Geometry check sheet. Reference: the model listing, model coordinates, mm. A direction names the side the tool comes from. Give positions to 0.01 mm unless a question says otherwise; leave off trailing zeros. Order: outer loops, then holes, each group sorted by start corner. A loop starts at its lowest first (then second) coordinate and runs counter-clockwise, first axis right, second up. Notation, with made-up numbers: M 21.5,6 L 48.5,6 A16 ccw 48.5,37 Z; hole C 46,66.25 d9. An arc over 180 degrees is marked long. Answer as CSV lines item,"result". Start each with the question number.
Q1. Set-up check for faces 1 (the flat face through (0, 3, 25)), 2 (the cylindrical face through (37.43, 0.6, -0.35)): record each of +Z, -Z, +X, -X, +Y, -Y from which the full face is reachable in a straight line by a thin tool's end or side.
Q2. Go/stop test with a flat-tipped pin: pin 1 (6 mm diameter, centred on x = -9, z = 21, fed in from +Y). Record where the tip stops, or that it passes through.
Q3. Section check D-D, the plane z = 0.5. Record the boundary of the cut face in (x, y), then the cut area to 3 significant figures.
Q4. Thickness scan on line 1 (X direction, y = 2.7, z = -23); line 2 (X direction, y = 3.25, z = -16); line 3 (Z direction, x = -3.5, y = 2.7). Record the ranges inside material, lowest first.
Q5. Section check C-C, the plane x = 25. Record the boundary of the cut face in (y, z), then the cut area to 3 significant figures.
Q6. Mould release check, pull along X, two halves, no side actions. Record for faces 3 (the cylindrical face through (37.43, 3.01, -26.4)), 4 (the cylindrical face through (0.5, 0.6, -26.43)), 5 (the flat face through (-1, 2, 0)): +X half, -X half, draft (parallel to the pull), parting line (faces both ways), or undercut.
Q7. Section check A-A, the plane z = -23. Record the boundary of the cut face in (x, y).
Q8. Section check B-B, the plane x = -34. Record the boundary of the cut face in (y, z), then the cut area to 3 significant figures.
```python
from build123d import *

# Parameters (mm, degrees)
SCHIZZO1_W                   = 76
SCHIZZO1_H                   = 54
ESTRUSIONE_ESTRUSIONE1_DEPTH = 4
SCHIZZO2_W                   = 72
SCHIZZO2_H                   = 50
TAGLIO_ESTRUSIONE1_DEPTH     = 2
SCHIZZO3_R                   = 3.65
SCHIZZO3_R_2                 = 1.65
ESTRUSIONE_ESTRUSIONE2_DEPTH = 2
SCHIZZO3_11_R                = 1.65
TAGLIO_ESTRUSIONE4_DEPTH     = 47.658332589
SCHIZZO5_R                   = 11
TAGLIO_ESTRUSIONE5_DEPTH     = 2
RACCORDO1_R                  = 2
RACCORDO2_R                  = 1


with BuildPart() as part:
    # Schizzo1 → Estrusione-Estrusione1 (new body)
    with BuildSketch(Plane(origin=(0, 0, 0), x_dir=(1, 0, 0), z_dir=(0, 1, 0))):
        Rectangle(SCHIZZO1_W, SCHIZZO1_H)
    extrude(amount=ESTRUSIONE_ESTRUSIONE1_DEPTH)

    # Schizzo2 → Taglio-Estrusione1 (cut)
    with BuildSketch(Plane(origin=(0, 4, 0), x_dir=(1, 0, 0), z_dir=(0, 1, 0))):
        Rectangle(SCHIZZO2_W, SCHIZZO2_H)
    extrude(amount=-TAGLIO_ESTRUSIONE1_DEPTH, mode=Mode.SUBTRACT)

    # Schizzo3 → Estrusione-Estrusione2 (add)
    # profile 1 of 4: a face of its own
    with BuildSketch(Plane(origin=(0, 2, 0), x_dir=(1, 0, 0), z_dir=(0, 1, 0))):
        with Locations((34, 23)):
            Circle(SCHIZZO3_R)
        with Locations(Location((34, 23, 0), (0, 0, 270))):
            Circle(SCHIZZO3_R_2, mode=Mode.SUBTRACT)
    # profile 2 of 4: a face of its own
    with BuildSketch(Plane(origin=(0, 2, 0), x_dir=(1, 0, 0), z_dir=(0, 1, 0))):
        with Locations((-34, 23)):
            Circle(SCHIZZO3_R)
        with Locations(Location((-34, 23, 0), (0, 0, 270))):
            Circle(SCHIZZO3_R_2, mode=Mode.SUBTRACT)
    # profile 3 of 4: a face of its own
    with BuildSketch(Plane(origin=(0, 2, 0), x_dir=(1, 0, 0), z_dir=(0, 1, 0))):
        with Locations((34, -23)):
            Circle(SCHIZZO3_R)
        with Locations(Location((34, -23, 0), (0, 0, 270))):
            Circle(SCHIZZO3_R_2, mode=Mode.SUBTRACT)
    # profile 4 of 4: a face of its own
    with BuildSketch(Plane(origin=(0, 2, 0), x_dir=(1, 0, 0), z_dir=(0, 1, 0))):
        with Locations((-34, -23)):
            Circle(SCHIZZO3_R)
        with Locations(Location((-34, -23, 0), (0, 0, 270))):
            Circle(SCHIZZO3_R_2, mode=Mode.SUBTRACT)
    extrude(amount=ESTRUSIONE_ESTRUSIONE2_DEPTH)

    # Schizzo3<11> → Taglio-Estrusione4 (cut, through all)
    with BuildSketch(Plane(origin=(0, 2, 0), x_dir=(1, 0, 0), z_dir=(0, 1, 0))):
        with Locations(Location((-34, 23, 0), (0, 0, 270))):
            Circle(SCHIZZO3_11_R)
        with Locations(Location((-34, -23, 0), (0, 0, 270))):
            Circle(SCHIZZO3_11_R)
        with Locations(Location((34, -23, 0), (0, 0, 270))):
            Circle(SCHIZZO3_11_R)
        with Locations(Location((34, 23, 0), (0, 0, 270))):
            Circle(SCHIZZO3_11_R)
    extrude(amount=-TAGLIO_ESTRUSIONE4_DEPTH, mode=Mode.SUBTRACT)

    # Schizzo5 → Taglio-Estrusione5 (cut)
    with BuildSketch(Plane.XZ):
        with Locations(Location((25, 8, 0), (0, 0, 270))):
            Circle(SCHIZZO5_R)
    extrude(amount=-TAGLIO_ESTRUSIONE5_DEPTH, mode=Mode.SUBTRACT)

    # Raccordo1
    raccordo1_edges = [part.edges().sort_by_distance(p)[0] for p in [
        (0, 0, 27),
        (-38, 0, 0),
        (0, 0, -27),
        (38, 0, 0),
        (38, 2, 27),
        (-38, 2, 27),
        (-38, 2, -27),
        (38, 2, -27),
    ]]
    fillet(raccordo1_edges, radius=RACCORDO1_R - 0.0001)  # a hair under: the kernel refuses the full size

    # Raccordo2
    raccordo2_edges = [part.edges().sort_by_distance(p)[0] for p in [
        (30.946723072, 3, -25),
        (36, 3, -19.946723072),
        (-36, 3, -19.946723072),
        (-30.946723072, 3, -25),
        (-30.946723072, 3, 25),
        (-36, 3, 19.946723072),
        (36, 3, 19.946723072),
        (30.946723072, 3, 25),
    ]]
    fillet(raccordo2_edges, radius=RACCORDO2_R)


solid = part.part
```
Answer block:
1,face 1,"+Y"
1,face 2,"+Z, -Z, +X, -Y"
2,pin 1,"stops at y = 2"
3,outline,"M -38,2 A2 ccw -36,0 L 16.95,0 L 16.95,2 L -36,2 L -36,4 L -38,4 Z; M 33.05,0 L 36,0 A2 ccw 38,2 L 38,4 L 36,4 L 36,2 L 33.05,2 Z"
3,area,"126 mm2"
4,line 1,"x = -38 to -35.65, -32.35 to -30.35, 30.35 to 32.35, 35.65 to 38"
4,line 2,"x = -38 to -36, 36 to 38"
4,line 3,"z = -27 to -25, 25 to 27"
5,outline,"M 0,-25 A2 ccw 2,-27 L 4,-27 L 4,-25 L 2,-25 L 2,-3 L 0,-3 Z; M 0,19 L 2,19 L 2,25 L 4,25 L 4,27 L 2,27 A2 ccw 0,25 Z"
5,area,"70.3 mm2"
6,face 3,"+X half"
6,face 4,"draft"
6,face 5,"undercut"
7,outline,"M -38,2 A2 ccw -36,0 L -35.65,0 L -35.65,4 L -38,4 Z; M -32.35,0 L 32.35,0 L 32.35,4 L 30.35,4 L 30.35,2 L -30.35,2 L -30.35,4 L -32.35,4 Z; M 35.65,0 L 36,0 A2 ccw 38,2 L 38,4 L 35.65,4 Z"
8,outline,"M 0,-25 A2 ccw 2,-27 L 4,-27 L 4,-24.65 L 0,-24.65 Z; M 0,-21.35 L 4,-21.35 L 4,-19.35 L 2,-19.35 L 2,19.35 L 4,19.35 L 4,21.35 L 0,21.35 Z; M 0,24.65 L 4,24.65 L 4,27 L 2,27 A2 ccw 0,25 Z"
8,area,"110 mm2"
